```python
from build123d import *

# Parameters (mm, degrees)
BOSS_EXTRUDE1_DEPTH = 23
SKETCH2_R           = 1.75
CUT_EXTRUDE1_DEPTH  = 11
SKETCH3_R           = 1.5
CUT_EXTRUDE2_DEPTH  = 10
SKETCH4_W           = 7
SKETCH4_H           = 5
BOSS_EXTRUDE2_DEPTH = 7
SKETCH5_R           = 3.75
SKETCH5_R_2         = 1.75
BOSS_EXTRUDE3_DEPTH = 5
SKETCH6_R           = 3.75
SKETCH6_R_2         = 1.75
BOSS_EXTRUDE4_DEPTH = 5
BOSS_EXTRUDE5_DEPTH = 5
BOSS_EXTRUDE6_DEPTH = 3.5
SKETCH9_W           = 5
SKETCH9_H           = 3
CUT_EXTRUDE3_DEPTH  = 20


with BuildPart() as part:
    # Sketch1 → Boss-Extrude1 (new body)
    with BuildSketch(Plane(origin=(0, 0, 0), x_dir=(1, 0, 0), z_dir=(0, 1, 0))):
        Polygon((0, 0), (-18, 0), (-22, 0), (-35, 0), (-35, -5), (-35, -10), (-15, -10), (-15, -5), (0, -5), align=None)
    extrude(amount=BOSS_EXTRUDE1_DEPTH)

    # Sketch2 → Cut-Extrude1 (cut, through all)
    with BuildSketch(Plane.XY.offset(10)):
        with Locations((-25, 16)):
            Circle(SKETCH2_R)
        with Locations((-4, 15)):
            Circle(SKETCH2_R)
    extrude(amount=-CUT_EXTRUDE1_DEPTH, mode=Mode.SUBTRACT)

    # Sketch3 → Cut-Extrude2 (cut)
    with BuildSketch(Plane.XZ):
        with Locations((-25, 2.5)):
            Circle(SKETCH3_R)
    extrude(amount=-CUT_EXTRUDE2_DEPTH, mode=Mode.SUBTRACT)

    # Sketch4 → Boss-Extrude2 (add)
    with BuildSketch(Plane.XZ):
        with Locations((-6.5, 2.5)):
            Rectangle(SKETCH4_W, SKETCH4_H)
    extrude(amount=BOSS_EXTRUDE2_DEPTH)

    # Sketch5 → Boss-Extrude3 (add)
    with BuildSketch(Plane.XY.offset(10)):
        with Locations((-25, 16)):
            Circle(SKETCH5_R)
        with Locations((-25, 16)):
            Circle(SKETCH5_R_2, mode=Mode.SUBTRACT)
    extrude(amount=BOSS_EXTRUDE3_DEPTH)

    # Sketch6 → Boss-Extrude4 (add)
    with BuildSketch(Plane.XY.offset(5)):
        with Locations((-4, 15)):
            Circle(SKETCH6_R)
        with Locations((-4, 15)):
            Circle(SKETCH6_R_2, mode=Mode.SUBTRACT)
    extrude(amount=BOSS_EXTRUDE4_DEPTH)

    # Sketch7 → Boss-Extrude5 (add)
    with BuildSketch(Plane.XY.offset(5)):
        Polygon((0, 0), (0, 23), (15.047232304, 23), (15.047232304, 15.047232304), align=None)
    extrude(amount=-BOSS_EXTRUDE5_DEPTH)

    # Sketch8 → Boss-Extrude6 (add)
    with BuildSketch(Plane.XY.offset(5)):
        Polygon((12.047232304, 23), (12.047232304, 16.289872991), (-1.242640687, 3), (-15, 3), (-15, 6), (-2.485281374, 6), (9.047232304, 17.532513678), (9.047232304, 23), align=None)
    extrude(amount=BOSS_EXTRUDE6_DEPTH)

    # Sketch9 → Cut-Extrude3 (cut)
    with BuildSketch(Plane(origin=(-15, 0, 0), x_dir=(0, 0, -1), z_dir=(1, 0, 0))):
        with Locations((-7.5, 1.5)):
            Rectangle(SKETCH9_W, SKETCH9_H)
    extrude(amount=-CUT_EXTRUDE3_DEPTH, mode=Mode.SUBTRACT)


solid = part.part
```
Geometry: final body of the model. Coordinates: model frame, mm. A direction names the side the tool comes from. Round coordinates to 2 decimals unless told otherwise and drop trailing zeros. Order: outer loops, then holes, each group sorted by start corner. A loop starts at its lowest first (then second) coordinate and runs counter-clockwise, first axis right, second up. Notation, with made-up numbers: (-3.75, -18) -> (10.25, -18) arc R25 ccw to (10.25, 15) -> close; hole circle Ø8 at (-36.5, 10.5). An arc over 180 degrees is marked (long way). Use one line per item in the form item = value. Start each with the question number.
1. Cut plane D-D (z = 9). Return the cut outline in (x, y).
2. Pin query (flat end, axial travel): pin 1 Ø16 at (x, y) = (3.5, 10) entering from +Z; pin 2 Ø4 at (x, z) = (-19, 3.5) entering from -Y; pin 3 Ø1.5 at (x, z) = (-25, 3) entering from -Y; pin 4 Ø2 at (x, y) = (-25, 16) entering from +Z. Return the tip coordinate at first contact, or that it passes through.
3. Reachability of faces 1 (the face through (-10, -3, 2)), 2 (the face through (-25, 10, 3)), 3 (the face through (-4.81, 11.34, 7.46)) from +Z, -Z, +X, -X, +Y, -Y: full face, straight path, thin tool, end or side. Return the list, or none.
4. Cut plane C-C (y = 0.75). Return the cut outline in (x, z), then the cut area to 3 significant figures.
5. Cut plane B-B (x = -4). Return the cut outline in (y, z), then the cut area to 3 significant figures.
6. Draft query along X for faces 4 (the face through (12.047, 20, 7)), 5 (the face through (-26.5, 4.93, 2.57)), 6 (the face through (-2, 14, 10)). Return one class per face: pulls with the +X half, pulls with the -X half, needs draft (parallel to the pull), parting line crosses it, or undercut.
7. Line query: probe 1 along Y at (x, z) = (-4, 6.35); probe 2 along Y at (x, z) = (-25, 8); probe 3 along X at (y, z) = (22.25, 7). Output: solid intervals per line, ascending.
8. Cut plane A-A (z = 6). Return the cut outline in (x, y), then the cut area to 3 significant figures.
Solution:
q1.outline = (-35, 3) -> (-15, 3) -> (-15, 23) -> (-35, 23) -> close; circle Ø7.5 at (-4, 15); hole circle Ø3.5 at (-25, 16); hole circle Ø3.5 at (-4, 15)
q2.pin_1 = 10
q2.pin_2 = 0
q2.pin_3 = 10
q2.pin_4 = through
q3.face_1 = +Z, -Z, -X, -Y
q3.face_2 = -Y
q3.face_3 = +Z
q4.outline = (-35, 0) -> (0.75, 0) -> (0.75, 5) -> (-35, 5) -> close; hole circle Ø3 at (-25, 2.5)
q4.area = 172 mm^2
q5.outline = (-7, 0) -> (13.25, 0) -> (13.25, 10) -> (11.25, 10) -> (11.25, 5) -> (6, 5) -> (6, 8.5) -> (3, 8.5) -> (3, 5) -> (-7, 5) -> close; (16.75, 0) -> (23, 0) -> (23, 5) -> (18.75, 5) -> (18.75, 10) -> (16.75, 10) -> close
q5.area = 163 mm^2
q6.face_4 = pulls with the +X half
q6.face_5 = undercut
q6.face_6 = needs draft
q7.probe_1 = 3 to 6, 11.25 to 13.25, 16.75 to 18.75
q7.probe_2 = 3 to 14.25, 17.75 to 23
q7.probe_3 = -35 to -15, 9.05 to 12.05
q8.outline = (-35, 3) -> (-1.24, 3) -> (12.05, 16.29) -> (12.05, 23) -> (9.05, 23) -> (9.05, 17.53) -> (-2.49, 6) -> (-15, 6) -> (-15, 23) -> (-35, 23) -> close; circle Ø7.5 at (-4, 15); hole circle Ø3.5 at (-25, 16); hole circle Ø3.5 at (-4, 15)
q8.area = 535 mm^2
